Check sheet for the modelled part. Datum: model origin and axes. Units: mm. A direction names the side the tool comes from. Round coordinates to 2 decimals unless told otherwise and drop trailing zeros. Write each loop counter-clockwise with the first axis right and the second up, starting at its lowest first coordinate (ties: lowest second). Pieces come first, ordered by that corner, then holes. Notation, with made-up numbers: M 86,-24.5 L 137,-24.5 A34 cw 137,7.5 Z; hole C -10.75,53 d3. An arc over 180 degrees is marked long. Answer in a Markdown table with one row per item.
Autodesk Fusion 360 part; units mm, degrees
sketch "Sketch1" plane through (0, 0, 0) normal (0, 0, 1) x (1, 0, 0)
  line L0 (0, 0) -> (0, 90)
  line L1 (0, 0) -> (90, 0)
  line L2 (0, 90) -> (20, 90)
  line L3 (90, 0) -> (90, 20)
  line L4 (90, 20) -> (70, 20)
  line L5 (20, 90) -> (20, 70)
  line L6 (20, 70) -> (70, 20)
  line L7 (10, 90) -> (10, 0) construction
  line L8 (90, 10) -> (0, 10) construction
  circle A0 centre (80, 10) radius 2.75
  circle A1 centre (25, 10) radius 2.75
  circle A2 centre (52.5, 10) radius 2.75
  line L9 (0, 0) -> (79.8876, 79.8876) construction
  line L10 (0, 0) -> (112.9781, 0) construction
  line L11 (25, 10) -> (52.5, 10) construction
  line L12 (52.5, 10) -> (80, 10) construction
  line L13 (45.75, 7) -> (31.75, 7)
  line L14 (31.75, 7) -> (31.75, 13)
  line L15 (31.75, 13) -> (45.75, 13)
  line L16 (45.75, 13) -> (45.75, 7)
  line L17 (45.75, 7) -> (31.75, 13) construction
  line L18 (31.75, 7) -> (45.75, 13) construction
  line L19 (73.25, 7) -> (59.25, 7)
  line L20 (59.25, 7) -> (59.25, 13)
  line L21 (59.25, 13) -> (73.25, 13)
  line L22 (73.25, 13) -> (73.25, 7)
  line L23 (73.25, 7) -> (59.25, 13) construction
  line L24 (59.25, 7) -> (73.25, 13) construction
  circle A3 centre (10, 25) radius 2.75
  line L25 (7, 31.75) -> (13, 31.75)
  line L26 (13, 31.75) -> (13, 45.75)
  line L27 (7, 45.75) -> (7, 31.75)
  line L28 (13, 45.75) -> (7, 45.75)
  line L29 (7, 59.25) -> (13, 59.25)
  line L30 (13, 59.25) -> (13, 73.25)
  line L31 (13, 73.25) -> (7, 73.25)
  line L32 (7, 73.25) -> (7, 59.25)
  circle A4 centre (10, 80) radius 2.75
  circle A5 centre (10, 52.5) radius 2.75
  point P0 (38.75, 10)
  point P1 (66.25, 10)
  dimension "d1" = 90
  dimension "d2" = 90
  dimension "d3" = 20
  dimension "d4" = 20
  dimension "d5" = 20
  dimension "d6" = 20
  dimension "d7" = 5.5
  dimension "d8" = 5.5
  dimension "d9" = 10
  dimension "d10" = 65
  dimension "d11" = 5.5
  dimension "d12" = 37.5
  dimension "d13" = 45
  dimension "d14" = 14
  dimension "d15" = 6
  dimension "d16" = 14
  dimension "d17" = 6
extrude "Extrude1" add sketch "Sketch1" along normal blind 4
extrude "Extrude3" add sketch "Sketch1" along normal blind 6 contours L13 L14 L15 L16 | L19 L20 L21 L22 | L25 L26 L27 L28 | L29 L30 L31 L32
sketch "Sketch2" plane through (0, 0, 4) normal (0, 0, 1) x (-1, 0, 0)
  circle A0 centre (-25, -10) radius 2.75
  circle A1 centre (-52.5, -10) radius 2.75
  circle A2 centre (-10, -80) radius 2.75
  circle A3 centre (-10, -25) radius 2.75
  circle A4 centre (-80, -10) radius 2.75
  circle A5 centre (-10, -52.5) radius 2.75
  line L0 (0, 0) -> (-90, 0)
  line L1 (-90, 0) -> (-90, -20)
  line L2 (-90, -20) -> (-70, -20)
  line L3 (-70, -20) -> (-20, -70)
  line L4 (-20, -70) -> (-20, -90)
  line L5 (-20, -90) -> (0, -90)
  line L6 (0, -90) -> (0, 0)
  line L7 (-20, -70) -> (-20, -20) construction
  line L8 (-20, -20) -> (-70, -20) construction
  line L9 (-20, -70) -> (-70, -20) construction
  line L10 (-23, -62.7574) -> (-62.7574, -23)
  line L11 (-23, -23) -> (-62.7574, -23)
  line L12 (-23, -62.7574) -> (-23, -23)
  line L13 (-7, -45.75) -> (-13, -45.75)
  line L14 (-13, -45.75) -> (-13, -31.75)
  line L15 (-13, -31.75) -> (-7, -31.75)
  line L16 (-7, -31.75) -> (-7, -45.75)
  line L17 (-59.25, -13) -> (-73.25, -13)
  line L18 (-73.25, -13) -> (-73.25, -7)
  line L19 (-73.25, -7) -> (-59.25, -7)
  line L20 (-59.25, -7) -> (-59.25, -13)
  line L21 (-7, -59.25) -> (-7, -73.25)
  line L22 (-7, -73.25) -> (-13, -73.25)
  line L23 (-13, -73.25) -> (-13, -59.25)
  line L24 (-13, -59.25) -> (-7, -59.25)
  line L25 (-31.75, -13) -> (-45.75, -13)
  line L26 (-45.75, -13) -> (-45.75, -7)
  line L27 (-45.75, -7) -> (-31.75, -7)
  line L28 (-31.75, -7) -> (-31.75, -13)
  dimension "d20" = 3
fillet "Fillet1" radius 5 7 edges at (0, 0, 2) (90, 0, 2) (90, 20, 2) (20, 70, 2) (70, 20, 2) (20, 90, 2) (0, 90, 2)
equation "d5 = d6"
1. Section check B-B, the plane y = 52.5. Record the cut outline in (x, z), and give its area (3 significant figures).
Found:
| item | result |
|---|---|
| outline | M 0,0 L 7.25,0 L 7.25,4 L 0,4 Z; M 12.75,0 L 37.5,0 L 37.5,4 L 12.75,4 Z |
| area | 128 mm2 |
2. Scan lines: L1, parallel to Y at x = 80, z = 1; L2, parallel to X at y = 10.5, z = 4.05; L3, parallel to Y at x = 10, z = 3.25. Record each from-to range of solid material in increasing order.
Found:
| item | result |
|---|---|
| L1 | y = 0 to 7.25, 12.75 to 20 |
| L2 | x = 31.75 to 45.75, 59.25 to 73.25 |
| L3 | y = 0 to 22.25, 27.75 to 49.75, 55.25 to 77.25, 82.75 to 90 |
3. Draft check along X on faces 6 (the face through (7, 66, 5)), 7 (the face through (70.13, 20.39, 2.03)), 8 (the face through (9.642, 49.773, 1.972)). Enter one of: +X half, -X half, draft (parallel to the pull), parting line (faces both ways), or undercut.
Found:
| item | result |
|---|---|
| face 6 | -X half |
| face 7 | +X half |
| face 8 | undercut |
4. Access from +Z, -Z, +X, -X, +Y, -Y to the whole of each face (thin tool, end or side, straight path). Record for faces 1 (the face through (31.75, 10, 5)), 2 (the face through (66, 13, 5)), 3 (the face through (66, 7, 5)), 4 (the face through (13, 66, 5)), 5 (the face through (39, 10, 6)).
Found:
| item | result |
|---|---|
| face 1 | +Z, -X, +Y, -Y |
| face 2 | +Z, +X, -X, +Y |
| face 3 | +Z, +X, -X, -Y |
| face 4 | +Z, +X, +Y, -Y |
| face 5 | +Z, +X, -X, +Y, -Y |
5. Section check C-C, the plane z = 3. Record the cut outline in (x, y).
Found:
| item | result |
|---|---|
| outline | M 0,5 A5 ccw 5,0 L 85,0 A5 ccw 90,5 L 90,15 A5 ccw 85,20 L 72.07,20 A5 cw 68.54,21.46 L 21.46,68.54 A5 cw 20,72.07 L 20,85 A5 ccw 15,90 L 5,90 A5 ccw 0,85 Z; hole C 10,25 d5.5; hole C 10,52.5 d5.5; hole C 10,80 d5.5; hole C 25,10 d5.5; hole C 52.5,10 d5.5; hole C 80,10 d5.5 |
6. Go/stop test with flat-tipped pins: pin 1 (1 mm diameter, centred on y = 75.5, z = 1.5, fed in from +X); pin 2 (0.6 mm diameter, centred on y = 10.5, z = 5.5, fed in from +X); pin 3 (3 mm diameter, centred on x = 26, z = 1, fed in from +Y); pin 4 (4.5 mm diameter, centred on x = 10, y = 52.5, fed in from -Z). Record where each tip stops, or that it passes through.
Found:
| item | result |
|---|---|
| pin 1 | stops at x = 20 |
| pin 2 | stops at x = 73.25 |
| pin 3 | stops at y = 65.5 |
| pin 4 | passes through |
7. Section check A-A, the plane x = 25. Record the cut outline in (y, z), and give its area (3 significant figures).
Found:
| item | result |
|---|---|
| outline | M 0,0 L 7.25,0 L 7.25,4 L 0,4 Z; M 12.75,0 L 65,0 L 65,4 L 12.75,4 Z |
| area | 238 mm2 |
8. Section check D-D, the plane y = 10. Record the cut outline in (x, z), and give its area (3 significant figures).
Found:
| item | result |
|---|---|
| outline | M 0,0 L 22.25,0 L 22.25,4 L 0,4 Z; M 27.75,0 L 49.75,0 L 49.75,4 L 45.75,4 L 45.75,6 L 31.75,6 L 31.75,4 L 27.75,4 Z; M 55.25,0 L 77.25,0 L 77.25,4 L 73.25,4 L 73.25,6 L 59.25,6 L 59.25,4 L 55.25,4 Z; M 82.75,0 L 90,0 L 90,4 L 82.75,4 Z |
| area | 350 mm2 |
